```python
from build123d import *

# Parameters (mm, degrees)
BOSS_EXTRUDE1_DEPTH = 186.944
CUT_EXTRUDE1_REACH  = 215.62
SKETCH2_R           = 11.1125
CUT_EXTRUDE2_REACH  = 207.171
SKETCH3_R           = 11.1125


with BuildPart() as part:
    # Sketch1 → Boss-Extrude1 (new body)
    with BuildSketch(Plane.XY):
        with BuildLine():
            Line((-47.62501925, 0), (-47.62501925, 76.2))
            ThreePointArc((-47.62501925, 76.2), (-43.134891189, 74.340128061), (-41.27501925, 69.85))
            Line((-41.27501925, 69.85), (-41.27501925, 14.2875))
            ThreePointArc((-41.27501925, 14.2875), (-38.950179326, 8.674839924), (-33.33751925, 6.35))
            Line((-33.33751925, 6.35), (22.22498075, 6.35))
            ThreePointArc((22.22498075, 6.35), (26.715108811, 4.490128061), (28.57498075, 0))
            Line((28.57498075, 0), (-47.62501925, 0))
        make_face()
    extrude(amount=-BOSS_EXTRUDE1_DEPTH)

    # Sketch2 → Cut-Extrude1 (cut, up to next)
    with BuildSketch(Plane(origin=(-41.27501925, 0, 0), x_dir=(0, 0, -1), z_dir=(1, 0, 0)), mode=Mode.PRIVATE) as cut_extrude1_sk1:
        with Locations((156.972, 42.06875)):
            Circle(SKETCH2_R)
    cut_extrude1_tool1 = extrude(cut_extrude1_sk1.sketch, amount=-CUT_EXTRUDE1_REACH, mode=Mode.PRIVATE) & part.part
    # Sketch2 → Cut-Extrude1 (cut, up to next)
    with BuildSketch(Plane(origin=(-41.27501925, 0, 0), x_dir=(0, 0, -1), z_dir=(1, 0, 0)), mode=Mode.PRIVATE) as cut_extrude1_sk2:
        with Locations((29.972, 42.06875)):
            Circle(SKETCH2_R)
    cut_extrude1_tool2 = extrude(cut_extrude1_sk2.sketch, amount=-CUT_EXTRUDE1_REACH, mode=Mode.PRIVATE) & part.part
    add(cut_extrude1_tool1.solids().sort_by_distance((-41.275019, 42.06875, -156.972))[0], mode=Mode.SUBTRACT)
    add(cut_extrude1_tool2.solids().sort_by_distance((-41.275019, 42.06875, -29.972))[0], mode=Mode.SUBTRACT)

    # Sketch3 → Cut-Extrude2 (cut, up to next)
    with BuildSketch(Plane(origin=(0, 6.35, 0), x_dir=(1, 0, 0), z_dir=(0, 1, 0)), mode=Mode.PRIVATE) as cut_extrude2_sk1:
        with Locations(Location((-5.55626925, 156.972, 0), (0, 0, 180))):
            Circle(SKETCH3_R)
    cut_extrude2_tool1 = extrude(cut_extrude2_sk1.sketch, amount=-CUT_EXTRUDE2_REACH, mode=Mode.PRIVATE) & part.part
    # Sketch3 → Cut-Extrude2 (cut, up to next)
    with BuildSketch(Plane(origin=(0, 6.35, 0), x_dir=(1, 0, 0), z_dir=(0, 1, 0)), mode=Mode.PRIVATE) as cut_extrude2_sk2:
        with Locations(Location((-5.55626925, 29.972, 0), (0, 0, 180))):
            Circle(SKETCH3_R)
    cut_extrude2_tool2 = extrude(cut_extrude2_sk2.sketch, amount=-CUT_EXTRUDE2_REACH, mode=Mode.PRIVATE) & part.part
    add(cut_extrude2_tool1.solids().sort_by_distance((-5.556269, 6.35, -156.972))[0], mode=Mode.SUBTRACT)
    add(cut_extrude2_tool2.solids().sort_by_distance((-5.556269, 6.35, -29.972))[0], mode=Mode.SUBTRACT)


solid = part.part
```
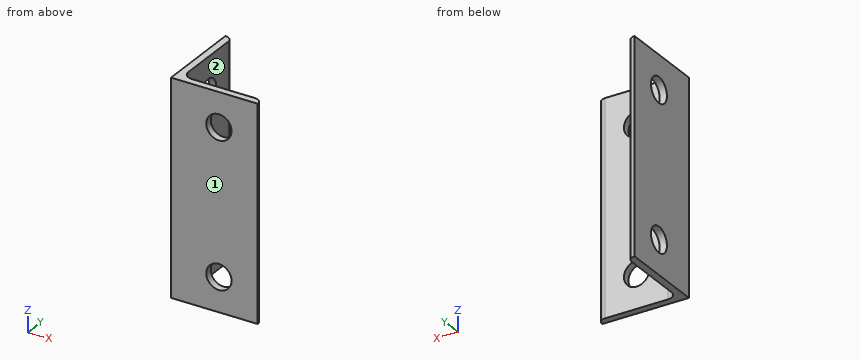
Can you work these out from the model? Positions are in its coordinate system, mm. Face numbers are marked on the shaded views. A direction names the side the tool comes from. Give positions to 0.01 mm unless a question says otherwise; leave off trailing zeros. Loops run counter-clockwise (first coordinate to the right, second up) from the corner with the lowest first, then second, coordinate; pieces in that order, holes last. Notation, with made-up numbers: M -21.75,28 L 37.25,28 A16 ccw 37.25,46 Z; hole C 89,53 d2. An arc over 180 degrees is marked long. Answer in a Markdown table with one row per item.
1. If I drill on line 1 along Y through (x, z) = (20, -100); line 2 along X through (y, z) = (55, -42); line 3 along Z through (x, y) = (4, 5), over which ranges is the centre line in solid material (lowest first)?
Taken from the geometry:
| item | result |
|---|---|
| line 1 | y = 0 to 6.35 |
| line 2 | x = -47.63 to -41.28 |
| line 3 | z = -186.94 to -162.64, -151.3 to -35.64, -24.3 to 0 |
2. Suppose I cut it at C-C on x = -4. Write out the boundary of the cut face in (y, z), plus the area to 3 significant figures.
Taken from the geometry:
| item | result |
|---|---|
| outline | M 0,-186.94 L 6.35,-186.94 L 6.35,-167.97 L 0,-167.97 Z; M 0,-145.97 L 6.35,-145.97 L 6.35,-40.97 L 0,-40.97 Z; M 0,-18.97 L 6.35,-18.97 L 6.35,0 L 0,0 Z |
| area | 908 mm² |
3. Suppose I cut it at B-B on y = 47.5. Write out the boundary of the cut face in (x, z), plus the area to 3 significant figures.
Taken from the geometry:
| item | result |
|---|---|
| outline | M -47.63,-186.94 L -41.28,-186.94 L -41.28,-166.67 L -47.63,-166.67 Z; M -47.63,-147.28 L -41.28,-147.28 L -41.28,-39.67 L -47.63,-39.67 Z; M -47.63,-20.28 L -41.28,-20.28 L -41.28,0 L -47.63,0 Z |
| area | 941 mm² |
4. For pin 1 Ø1.5 at (x, z) = (3, -49.5) entering from +Y; pin 2 Ø1 at (y, z) = (24.5, -157) entering from +X (3 decimals); pin 3 Ø6 at (y, z) = (11.5, -21) entering from +X, each with a flat end and sliding along its axis, tell me the tip position at first contact or that it passes through.
Taken from the geometry:
| item | result |
|---|---|
| pin 1 | stops at y = 6.35 |
| pin 2 | stops at x = -41.275 |
| pin 3 | stops at x = -38.77 |
5. Suppose I cut it at A-A on z = -153. Count the separate pieces of the cut face and the enclosed holes in it, plus the area to 3 significant figures.
Taken from the geometry:
| item | result |
|---|---|
| separate pieces | 3 |
| enclosed holes | 0 |
| area | 660 mm² |
6. Which directions (+Z, -Z, +X, -X, +Y, -Y) give clear straight access to the entire face, cutting with the end or side of a thin tool? Please do the marked faces 1 and 2.
Taken from the geometry:
| item | result |
|---|---|
| face 1 | +Z, -Z, +X, -X, -Y |
| face 2 | +Z, -Z, +X, +Y |
